Build history of the part. All positions in model axes, mm. A direction names the side the tool comes from. Round coordinates to 2 decimals unless told otherwise and drop trailing zeros. Write each loop counter-clockwise with the first axis right and the second up, starting at its lowest first coordinate (ties: lowest second). Pieces come first, ordered by that corner, then holes. Notation, with made-up numbers: (80, 12.5) -> (136, 12.5) arc R34 cw to (136, 48.5) -> close; hole circle Ø4 at (-38.5, 80). An arc over 180 degrees is marked (long way). Return JSON: item names as keys, results as strings.
Autodesk Inventor part; units mm, degrees
ref_plane "Plano de trabajo1" through (-37.5, 25, -15) normal (0, -0.866, -0.5) x (1, 0, 0)
ref_plane "YZ Plane" through (0, 0, 0) normal (1, 0, 0) x (0, 1, 0)
ref_plane "XZ Plane" through (0, 0, 0) normal (0, 1, 0) x (-1, 0, 0)
sketch "Boceto1" plane through (0, 0, 0) normal (0, 1, 0) x (-1, 0, 0)
  line L0 (-37.5, -50) -> (37.5, -50)
  line L1 (37.5, -50) -> (37.5, 50)
  line L2 (37.5, 50) -> (-37.5, 50)
  line L3 (-37.5, 50) -> (-37.5, -50)
  line L4 (-37.5, -50) -> (37.5, 50) construction
  line L5 (37.5, -50) -> (-37.5, 50) construction
  line L6 (37.5, 50) -> (7.5, 50)
  line L7 (7.5, 50) -> (7.5, 15)
  line L8 (7.5, 15) -> (37.5, 15)
  line L9 (37.5, 15) -> (37.5, 50)
  point P0 (0, 0)
  dimension "d0" = 100
  dimension "d1" = 75
  dimension "d2" = 30
  dimension "d3" = 35
extrude "Extrusión1" add sketch "Boceto1" along normal blind 15 contours L3 L2 L7 L8 L1 L0
sketch "Boceto2" plane through (0, 15, 0) normal (0, 1, 0) x (1, 0, 0)
  line L0 (-37.5, 50) -> (-37.5, -15)
  line L1 (-37.5, 50) -> (37.5, 50)
  line L2 (37.5, 50) -> (37.5, 15)
  line L3 (37.5, 15) -> (-37.5, 15)
  line L4 (-37.5, 15) -> (-37.5, 50)
  point P0 (0, 0)
  dimension "d6" = 35
  dimension "d7" = 75
extrude "Extrusión2" add sketch "Boceto2" along normal blind 10
ref_plane "Plano de trabajo1" through (-37.5, 25, -15) normal (0, -0.866, -0.5) x (1, 0, 0)
sketch "Boceto3" plane through (-37.5, 25, -15) normal (0, -0.866, -0.5) x (1, 0, 0)
  line L0 (75, 5) -> (75, 0)
  line L1 (75, 0) -> (50, 0)
  line L2 (0, 0) -> (75, 0)
  line L3 (0, 30.9808) -> (30, 30.9808)
  line L4 (0, 5) -> (0, 0)
  line L5 (0, 30.9808) -> (0, 0)
  arc A0 (0, 0) -> (50, 0) centre (25, 0) ccw
  line L6 (50, 0) -> (50, 30.9808)
  line L7 (50, 30.9808) -> (0, 30.9808)
  circle A1 centre (25, 0) radius 10
  point P0 (37.5, 25.4904)
  point P1 (0, 5)
  dimension "d11" = 25
  dimension "d12" = 20
extrude "Extrusión3" add sketch "Boceto3" along normal blind 10 contours A1 L2 L4 L5 L3 L7 L6 | L2 A0 A1
sketch "Boceto4" plane through (-37.5, 25, -15) normal (0, 0.866, 0.5) x (1, 0, 0)
  line L0 (15, 0) -> (35, 0)
  circle A0 centre (25, 0) radius 10
  point P0 (37.5, -25.4904)
  dimension "d15" = 20
extrude "Extrusión4" cut sketch "Boceto4" against normal blind 40
sketch "Boceto5" plane through (37.5, 0, 50) normal (1, 0, 0) x (0, 0, -1)
  line L0 (35, 15) -> (0, 15)
  line L1 (0, 15) -> (0, 10)
  line L2 (0, 0) -> (0, 15)
  line L3 (0, 10) -> (69.9738, 10)
  line L4 (100, 0) -> (100, 25)
  line L5 (65, 25) -> (47.6795, 15)
  line L6 (65, 15) -> (65, 25)
  arc A0 (62.0755, 49.9347) -> (65, 25) centre (41.9437, 34.9347) ccw
  circle A1 centre (41.9437, 34.9347) radius 25.1056
  line L7 (0, 15) -> (65, 15)
  circle A2 centre (41.9437, 34.9347) radius 30.4793
  line L8 (65, 25) -> (70.7584, 25)
  line L9 (65, 25) -> (100, 25)
  point P0 (50, 0)
  point P1 (57.2047, 15)
  point P2 (62.0755, 49.9347)
  point P3 (39.0192, 10)
  point P4 (44.8682, 10)
  dimension "d18" = 5
extrude "Extrusión5" add sketch "Boceto5" against normal blind 25 contours L7 A0 L3 L0 | L0 A0 A1 L5 L7 | L5 A0 L7 | L6 L7 A0
sketch "Boceto6" plane through (37.5, 0, 50) normal (1, 0, 0) x (0, 0, -1)
  arc A0 (65, 25) -> (26.6827, 15) centre (41.9437, 34.9347) ccw
  circle A1 centre (41.9437, 34.9347) radius 25.1056
  point P0 (50, 0)
  point P1 (26.6827, 15)
extrude "Extrusión6" cut sketch "Boceto6" against normal blind 25
sketch "Boceto7" plane through (-37.5, 25, -15) normal (0, -0.866, -0.5) x (1, 0, 0)
  point P0 (37.5, 25.4904)
sketch "Boceto8" plane through (0, 25, 0) normal (0, 1, 0) x (1, 0, 0)
  circle A0 centre (22.5, 35) radius 5
  line L0 (37.5, 50) -> (-37.5, 50)
  line L1 (37.5, 15) -> (37.5, 50)
  circle A1 centre (22.5, -40) radius 5
  line L2 (-7.5, -50) -> (37.5, -50)
  line L3 (37.5, -50) -> (37.5, -23.3173)
  point P0 (0, 0)
  dimension "d23" = 15
  dimension "d24" = 15
  dimension "d25" = 10
  dimension "d26" = 10
  dimension "d27" = 15
  dimension "d28" = 10
extrude "Extrusión7" cut sketch "Boceto8" against normal blind 25
properties part number "Pieza3-Tarea2"
Q1. Pin check, flat tips, straight feed: pin 1 Ø2 at (x, z) = (-9, -35.5) entering from -Y; pin 2 Ø4 at (x, z) = (21.5, 35.5) entering from +Y; pin 3 Ø6 at (x, z) = (22.5, 40) entering from -Y; pin 4 Ø6 at (x, z) = (26.5, -26) entering from +Y. Stop position of each tip, or through.
Verdict:
{"pin 1": "stops at y = 6.32", "pin 2": "stops at y = 15", "pin 3": "passes through", "pin 4": "stops at y = 25"}
Q2. Wall check: L1, parallel to Z at x = 22, y = 3; L2, parallel to X at y = 10.5, z = 40; L3, parallel to X at y = 15, z = -35. Give the ranges that are in metal, low to high.
Verdict:
{"L1": "z = -50 to -39.97, -30.03 to 35.03, 44.97 to 50", "L2": "x = -7.5 to 17.5, 27.5 to 37.5", "L3": "x = -37.5 to 17.5, 27.5 to 37.5"}
Q3. Saw through at B-B on z = 40. List the corners of the cut face in (x, y), then the cut area to 3 significant figures.
Verdict:
{"outline": "(-7.5, 0) -> (17.5, 0) -> (17.5, 15) -> (-7.5, 15) -> close; (27.5, 0) -> (37.5, 0) -> (37.5, 15) -> (27.5, 15) -> close", "area": "525 mm²"}
Q4. Two-plate mould, pull along Z, no slides. Class faces 6 (the flat face through (-22, 7, 15)), 7 (the flat face through (37.5, 10, -10)), 8 (the cylindrical face through (25.175, 10.564, 2.026)): +Z half, -Z half, draft (parallel to the pull), parting line (faces both ways), or undercut.
Verdict:
{"face 6": "+Z half", "face 7": "draft", "face 8": "undercut"}
Q5. 3-axis set-ups, long thin cutter, end or side, ignore diameter. For faces 1 (the flat face through (-37.5, 12, -18)), 2 (the flat face through (12.5, 14.6, 2.8)), 3 (the flat face through (9, 15, 26)), 4 (the flat face through (-7.5, 7, 33)), 5 (the cylindrical face through (-11.95, 34.19, -38.555)): which of +Z, -Z, +X, -X, +Y, -Y reach the whole face in a straight line?
Verdict:
{"face 1": "+Z, -Z, -X, +Y, -Y", "face 2": "+X, +Y", "face 3": "+Z, +X, -X, +Y", "face 4": "+Z, -X, +Y, -Y", "face 5": "-Z, +Y"}
Q6. Saw through at C-C on x = -15.5. List the corners of the cut face in (y, z).
Verdict:
{"outline": "(0, -50) -> (25, -50) -> (25, -35) -> (28.75, -41.49) -> (37.41, -36.49) -> (29.77, -23.26) -> (0, -40.45) -> close; (0, -18.42) -> (20.23, -6.74) -> (15, 2.32) -> (15, 15) -> (0, 15) -> close"}
Q7. Saw through at D-D on z = 26. List the corners of the cut face in (x, y).
Verdict:
{"outline": "(-7.5, 0) -> (37.5, 0) -> (37.5, 15) -> (-7.5, 15) -> close"}
Q8. Saw through at A-A on x = 22.5. List the corners of the cut face in (y, z).
Verdict:
{"outline": "(0, -50) -> (25, -50) -> (25, -40) -> (0, -40) -> close; (0, -30) -> (25, -30) -> (25, -15) arc R25.11 cw to (15, 23.32) -> (15, 35) -> (0, 35) -> close; (0, 45) -> (15, 45) -> (15, 50) -> (0, 50) -> close"}
